Geometry: final body of the model. Coordinates: model frame, mm. Face numbers are marked on the shaded views. Round coordinates to 2 decimals unless told otherwise and drop trailing zeros. Loops run counter-clockwise (first coordinate to the right, second up) from the corner with the lowest first, then second, coordinate; pieces in that order, holes last. Notation, with made-up numbers: (8.25, 22) - (67.25, 22) arc R22 cw to (67.25, 43) - close; hole circle Ø9 at (81, -18.5). An arc over 180 degrees is marked (long way). Return JSON: item names as keys, results as strings. Group by question number.
1. Section B-B on y = 11.75. Return loops of the section in (x, z).
2. Material intervals for probe 1 along X at (y, z) = (1.1, 42); probe 2 along X at (y, z) = (7.25, 106.5); probe 3 along Y at (x, z) = (8.5, 19.5), sorted ascending.
3. First-contact query: pin 1 Ø9.5 at (x, z) = (15, 138) entering from -Y; pin 2 Ø11.5 at (x, z) = (15, 26) entering from +Y; pin 3 Ø1.5 at (y, z) = (6.5, 145) entering from +X. Flat tips, straight axial feed; report the tip coordinate or a pass-through.
4. Section D-D on z = 111.5. Return loops of the section in (x, y), and give its area (3 significant figures).
5. Draft query along X for the marked faces 1, 2, 3 and 4. Return one class per face: +X half, -X half, draft (parallel to the pull), parting line (faces both ways), or undercut.
6. Section A-A on x = 15. Return loops of the section in (y, z).
7. Section C-C on z = 138. Return loops of the section in (x, y), and give its area (3 significant figures).
from build123d import *

# Parameters (mm, degrees)
P_IDAT_VYSUNUT_M1_DEPTH  = 180
ODEBRAT_VYSUNUT_M1_REACH = 4
SKICA2_R                 = 3
SKICA2_R_2               = 4.5
ODEBRAT_VYSUNUT_M2_DEPTH = 15


with BuildPart() as part:
    # Skica1 → Přidat vysunutím1 (new body)
    with BuildSketch(Plane.XY):
        Polygon((28, 15), (30, 15), (30, 0), (0, 0), (0, 15), (2, 15), (2, 2), (28, 2), align=None)
    extrude(amount=P_IDAT_VYSUNUT_M1_DEPTH)

    # Skica2 → Odebrat vysunutím1 (cut, up to next)
    with BuildSketch(Plane(origin=(0, 2, 0), x_dir=(1, 0, 0), z_dir=(0, 1, 0)), mode=Mode.PRIVATE) as odebrat_vysunut_m1_sk1:
        with Locations((15, -170)):
            Circle(SKICA2_R)
    odebrat_vysunut_m1_tool1 = extrude(odebrat_vysunut_m1_sk1.sketch, amount=-ODEBRAT_VYSUNUT_M1_REACH, mode=Mode.PRIVATE) & part.part
    add(odebrat_vysunut_m1_tool1.solids().sort_by_distance((15, 2, 170))[0], mode=Mode.SUBTRACT)
    # Skica2 → Odebrat vysunutím1 (cut, up to next)
    with BuildSketch(Plane(origin=(0, 2, 0), x_dir=(1, 0, 0), z_dir=(0, 1, 0)), mode=Mode.PRIVATE) as odebrat_vysunut_m1_sk2:
        with Locations((15, -154)):
            Circle(SKICA2_R_2)
    odebrat_vysunut_m1_tool2 = extrude(odebrat_vysunut_m1_sk2.sketch, amount=-ODEBRAT_VYSUNUT_M1_REACH, mode=Mode.PRIVATE) & part.part
    add(odebrat_vysunut_m1_tool2.solids().sort_by_distance((15, 2, 154))[0], mode=Mode.SUBTRACT)
    # Skica2 → Odebrat vysunutím1 (cut, up to next)
    with BuildSketch(Plane(origin=(0, 2, 0), x_dir=(1, 0, 0), z_dir=(0, 1, 0)), mode=Mode.PRIVATE) as odebrat_vysunut_m1_sk3:
        with Locations((15, -138)):
            Circle(SKICA2_R)
    odebrat_vysunut_m1_tool3 = extrude(odebrat_vysunut_m1_sk3.sketch, amount=-ODEBRAT_VYSUNUT_M1_REACH, mode=Mode.PRIVATE) & part.part
    add(odebrat_vysunut_m1_tool3.solids().sort_by_distance((15, 2, 138))[0], mode=Mode.SUBTRACT)
    # Skica2 → Odebrat vysunutím1 (cut, up to next)
    with BuildSketch(Plane(origin=(0, 2, 0), x_dir=(1, 0, 0), z_dir=(0, 1, 0)), mode=Mode.PRIVATE) as odebrat_vysunut_m1_sk4:
        with Locations((15, -42)):
            Circle(SKICA2_R)
    odebrat_vysunut_m1_tool4 = extrude(odebrat_vysunut_m1_sk4.sketch, amount=-ODEBRAT_VYSUNUT_M1_REACH, mode=Mode.PRIVATE) & part.part
    add(odebrat_vysunut_m1_tool4.solids().sort_by_distance((15, 2, 42))[0], mode=Mode.SUBTRACT)
    # Skica2 → Odebrat vysunutím1 (cut, up to next)
    with BuildSketch(Plane(origin=(0, 2, 0), x_dir=(1, 0, 0), z_dir=(0, 1, 0)), mode=Mode.PRIVATE) as odebrat_vysunut_m1_sk5:
        with Locations((15, -26)):
            Circle(SKICA2_R_2)
    odebrat_vysunut_m1_tool5 = extrude(odebrat_vysunut_m1_sk5.sketch, amount=-ODEBRAT_VYSUNUT_M1_REACH, mode=Mode.PRIVATE) & part.part
    add(odebrat_vysunut_m1_tool5.solids().sort_by_distance((15, 2, 26))[0], mode=Mode.SUBTRACT)
    # Skica2 → Odebrat vysunutím1 (cut, up to next)
    with BuildSketch(Plane(origin=(0, 2, 0), x_dir=(1, 0, 0), z_dir=(0, 1, 0)), mode=Mode.PRIVATE) as odebrat_vysunut_m1_sk6:
        with Locations((15, -10)):
            Circle(SKICA2_R)
    odebrat_vysunut_m1_tool6 = extrude(odebrat_vysunut_m1_sk6.sketch, amount=-ODEBRAT_VYSUNUT_M1_REACH, mode=Mode.PRIVATE) & part.part
    add(odebrat_vysunut_m1_tool6.solids().sort_by_distance((15, 2, 10))[0], mode=Mode.SUBTRACT)

    # Skica3 → Odebrat vysunutím2 (cut)
    with BuildSketch(Plane.XZ):
        Polygon((30, 180), (20, 180), (30, 140), align=None)
        Polygon((0, 0), (10, 0), (0, 40), align=None)
        Polygon((10, 180), (0, 140), (0, 180), align=None)
        Polygon((20, 0), (30, 40), (30, 0), align=None)
    extrude(amount=-ODEBRAT_VYSUNUT_M2_DEPTH, mode=Mode.SUBTRACT)


solid = part.part
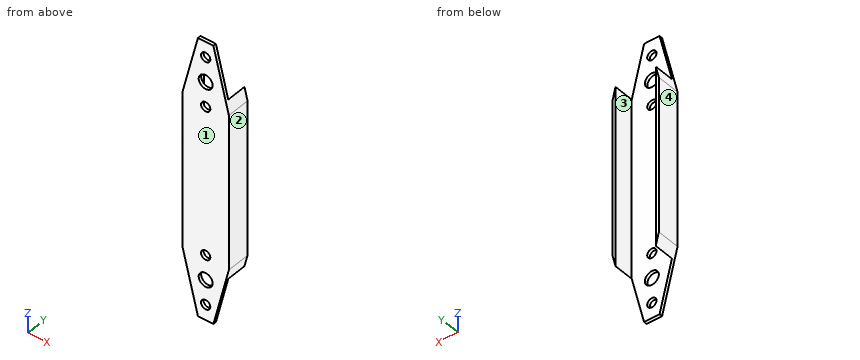
Taken from the geometry:
{
 "1": {"outline": "(0, 40) - (2, 32) - (2, 148) - (0, 140) - close; (28, 32) - (30, 40) - (30, 140) - (28, 148) - close"},
 "2": {"probe 1": "0 to 12, 18 to 30", "probe 2": "0 to 2, 28 to 30", "probe 3": "0 to 2"},
 "3": {"pin 1": "y = 0", "pin 2": "y = 2", "pin 3": "x = 28.94"},
 "4": {"outline": "(0, 0) - (30, 0) - (30, 15) - (28, 15) - (28, 2) - (2, 2) - (2, 15) - (0, 15) - close", "area": "112 mm2"},
 "5": {"face 1": "draft", "face 2": "+X half", "face 3": "undercut", "face 4": "-X half"},
 "6": {"outline": "(0, 0) - (2, 0) - (2, 7) - (0, 7) - close; (0, 13) - (2, 13) - (2, 21.5) - (0, 21.5) - close; (0, 30.5) - (2, 30.5) - (2, 39) - (0, 39) - close; (0, 45) - (2, 45) - (2, 135) - (0, 135) - close; (0, 141) - (2, 141) - (2, 149.5) - (0, 149.5) - close; (0, 158.5) - (2, 158.5) - (2, 167) - (0, 167) - close; (0, 173) - (2, 173) - (2, 180) - (0, 180) - close"},
 "7": {"outline": "(0, 0) - (12, 0) - (12, 2) - (2, 2) - (2, 15) - (0, 15) - close; (18, 0) - (30, 0) - (30, 15) - (28, 15) - (28, 2) - (18, 2) - close", "area": "100 mm2"}
}
